Solid Edge part; units mm, degrees
sketch "Sketch1" plane through (0, 0, 0) normal (0, 0, 1) x (1, 0, 0)
  circle A0 centre (0, 0) radius 31.242
extrude "Protrusion1" add sketch "Sketch1" along normal blind 3.175
hole "Hole_1" at (0, 0, 3.175) direction (0, 0, -1) diameter 9.525 end up to next
hole "Hole_2" at (5.6127, 5.6127, 3.175) direction (0, 0, -1) diameter 3.5052 end up to next
hole "Hole1" at (5.6127, -5.6127, 3.175) direction (0, 0, -1) diameter 3.5052 end up to next
hole "Hole2" at (-5.6127, -5.6127, 3.175) direction (0, 0, -1) diameter 3.5052 end up to next
hole "Hole3" at (-5.6127, 5.6127, 3.175) direction (0, 0, -1) diameter 3.5052 end up to next
properties part number "ARM-04" material "Polypropylene, general purpose"
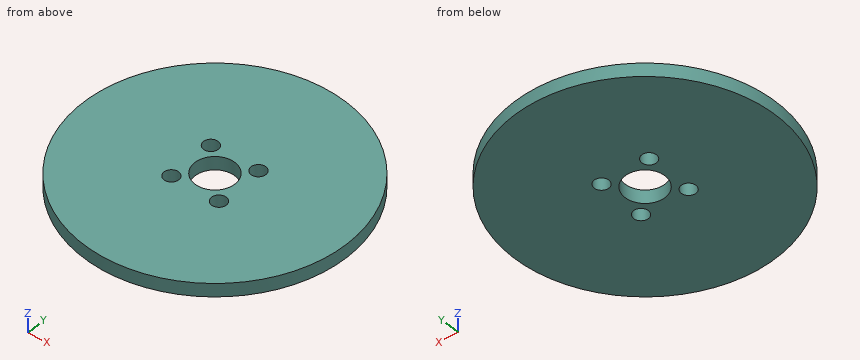
Source: CAD feature listing. Evaluate the final solid. Frame: model axes, mm. Round coordinates to 2 decimals unless told otherwise and drop trailing zeros. Loops run counter-clockwise (first coordinate to the right, second up) from the corner with the lowest first, then second, coordinate; pieces in that order, holes last. Notation, with made-up numbers: (8.5, -4) - (65.5, -4) arc R8 cw to (65.5, 6) - close; hole circle Ø7 at (41.5, -6). An arc over 180 degrees is marked (long way). Write item = value, one per line. Start each with the question number.
Item 1: Section query D-D on x = 22. Output: boundary loops of the cut face in (y, z) (3 decimals), plus the area to 3 significant figures.
Item 2: Section query C-C on z = 1.6. Output: boundary loops of the cut face in (x, y) (1 decimal).
Item 3: Material intervals for line 1 (X direction, y = 5.5, z = 2.55); line 2 (Y direction, x = -7, z = 2.35); line 3 (Y direction, x = 0, z = 0.7), sorted ascending.
Item 4: Section query A-A on x = 0. Output: boundary loops of the cut face in (y, z) (1 decimal).
Results list:
q1.outline = (-22.182, 0) - (22.182, 0) - (22.182, 3.175) - (-22.182, 3.175) - close
q1.area = 141 mm²
q2.outline = circle Ø62.5 at (0, 0); hole circle Ø3.5 at (-5.6, -5.6); hole circle Ø3.5 at (-5.6, 5.6); hole circle Ø9.5 at (0, 0); hole circle Ø3.5 at (5.6, -5.6); hole circle Ø3.5 at (5.6, 5.6)
q3.line_1 = -30.75 to -7.36, -3.86 to 3.86, 7.36 to 30.75
q3.line_2 = -30.45 to -6.68, -4.54 to 4.54, 6.68 to 30.45
q3.line_3 = -31.24 to -4.76, 4.76 to 31.24
q4.outline = (-31.2, 0) - (-4.8, 0) - (-4.8, 3.2) - (-31.2, 3.2) - close; (4.8, 0) - (31.2, 0) - (31.2, 3.2) - (4.8, 3.2) - close
